```python
from build123d import *

# Parameters (mm, degrees)
SKETCH_1_R          = 3.2
SKETCH_1_R_2        = 3
SKETCH_1_W          = 46
SKETCH_1_H          = 34
EXTRUDE_1_DEPTH     = 13
SKETCH_2_R          = 11.4
EXTRUDE_2_DEPTH     = 14
SKETCH_3_R          = 1.25
CUT_EXTRUDE_1_DEPTH = 11
CUT_EXTRUDE_2_DEPTH = 14
SKETCH_5_R          = 4
EXTRUDE_3_DEPTH     = 2
SKETCH_6_R          = 1.5
EXTRUDE_4_DEPTH     = 5
EXTRUDE_5_DEPTH     = 1
SKETCH_9_W          = 26.5
SKETCH_9_H          = 7.251384336
CUT_EXTRUDE_4_DEPTH = 10


with BuildPart() as part:
    # 스케치1 → 보스-돌출1 (new body)
    with BuildSketch(Plane(origin=(0, 0, 0), x_dir=(1, 0, 0), z_dir=(0, 1, 0))):
        with BuildLine():
            Line((-61.498388188, 66.010476517), (61.501611812, 65.989522963))
            ThreePointArc((61.501611812, 65.989522963), (65.036624731, 64.524771992), (66.500805906, 60.989523028))
            Line((66.500805906, 60.989523028), (66.500805906, 4.989523158))
            ThreePointArc((66.500805906, 4.989523158), (65.03605487, 1.453704333), (61.5, -0.010476777))
            Line((61.5, -0.010476777), (-61.5, 0.010476777))
            ThreePointArc((-61.5, 0.010476777), (-65.035012919, 1.475227749), (-66.499194094, 5.010476712))
            Line((-66.499194094, 5.010476712), (-66.499194094, 61.010476582))
            ThreePointArc((-66.499194094, 61.010476582), (-65.034443058, 64.546295408), (-61.498388188, 66.010476517))
        make_face()
        with Locations((-19.054194094, 45.730282553)):
            Circle(SKETCH_1_R, mode=Mode.SUBTRACT)
        with Locations((-24.324694094, 40.396282553)):
            Circle(SKETCH_1_R, mode=Mode.SUBTRACT)
        with Locations((-13.783694094, 40.396282553)):
            Circle(SKETCH_1_R, mode=Mode.SUBTRACT)
        with Locations((-19.054194094, 35.062282553)):
            Circle(SKETCH_1_R, mode=Mode.SUBTRACT)
        with Locations((-17.339694094, 58.303282553)):
            Circle(SKETCH_1_R_2, mode=Mode.SUBTRACT)
        with Locations((43.112305906, 58.303282553)):
            Circle(SKETCH_1_R_2, mode=Mode.SUBTRACT)
        with Locations((50.675805906, 42.811282553)):
            Circle(SKETCH_1_R_2, mode=Mode.SUBTRACT)
        with Locations((43.048805906, 37.919782553)):
            Circle(SKETCH_1_R_2, mode=Mode.SUBTRACT)
        with Locations((15.743805906, 36.713282553)):
            Rectangle(SKETCH_1_W, SKETCH_1_H, mode=Mode.SUBTRACT)
    extrude(amount=EXTRUDE_1_DEPTH)

    # 스케치2 → 보스-돌출2 (add)
    with BuildSketch(Plane(origin=(0, 13, 0), x_dir=(1, 0, 0), z_dir=(0, 1, 0))):
        with BuildLine():
            ThreePointArc((-59.454194094, 37.696962121), (-55.060795812, 27.090360404), (-44.454194094, 22.696962121))
            ThreePointArc((-44.454194094, 22.696962121), (-33.847592376, 27.090360404), (-29.454194094, 37.696962121))
            Line((-29.454194094, 37.696962121), (-29.454194094, 41.666282553))
            ThreePointArc((-29.454194094, 41.666282553), (-44.454194094, 56.666282553), (-59.454194094, 41.666282553))
            Line((-59.454194094, 41.666282553), (-59.454194094, 37.696962121))
        make_face()
        with Locations((-44.454194094, 41.666282553)):
            Circle(SKETCH_2_R, mode=Mode.SUBTRACT)
    extrude(amount=EXTRUDE_2_DEPTH)

    # 스케치3 → 컷-돌출1 (cut)
    with BuildSketch(Plane.XZ):
        with Locations((-60.440145734, -59.928842317)):
            Circle(SKETCH_3_R)
        with Locations((-60.440145734, -6.092110978)):
            Circle(SKETCH_3_R)
        with Locations((60.442726529, -59.928842317)):
            Circle(SKETCH_3_R)
        with Locations((60.442726529, -6.092110978)):
            Circle(SKETCH_3_R)
        with BuildLine():
            Line((-56.500826452, -64.009622683), (56.500826452, -63.990377307))
            Line((56.500826452, -63.990377307), (56.500826452, -60.989502488))
            ThreePointArc((56.500826452, -60.989502488), (57.965286528, -57.453983111), (61.500805906, -55.989523034))
            Line((61.500805906, -55.989523034), (64.500805906, -55.989523034))
            Line((64.500805906, -55.989523034), (64.500805906, -9.989482066))
            Line((64.500805906, -9.989482066), (61.500805906, -9.989482066))
            ThreePointArc((61.500805906, -9.989482066), (57.965286528, -8.52502199), (56.500826452, -4.989502612))
            Line((56.500826452, -4.989502612), (56.500826452, -1.990377339))
            Line((56.500826452, -1.990377339), (-56.500826452, -2.009622715))
            Line((-56.500826452, -2.009622715), (-56.500826452, -4.989502612))
            ThreePointArc((-56.500826452, -4.989502612), (-57.965286528, -8.52502199), (-61.500805906, -9.989482066))
            Line((-61.500805906, -9.989482066), (-64.499194094, -9.989482066))
            Line((-64.499194094, -9.989482066), (-64.499194094, -55.989523034))
            Line((-64.499194094, -55.989523034), (-61.500805906, -55.989523034))
            ThreePointArc((-61.500805906, -55.989523034), (-57.965286528, -57.453983111), (-56.500826452, -60.989502488))
            Line((-56.500826452, -60.989502488), (-56.500826452, -64.009622683))
        make_face()
    extrude(amount=-CUT_EXTRUDE_1_DEPTH, mode=Mode.SUBTRACT)

    # 스케치4 → 컷-돌출2 (cut)
    with BuildSketch(Plane.XZ.offset(-11)):
        with BuildLine():
            Line((-31.454194094, -41.666282553), (-31.454194094, -37.696962121))
            ThreePointArc((-31.454194094, -37.696962121), (-35.261805939, -28.504573966), (-44.454194094, -24.696962121))
            ThreePointArc((-44.454194094, -24.696962121), (-53.646582249, -28.504573966), (-57.454194094, -37.696962121))
            Line((-57.454194094, -37.696962121), (-57.454194094, -41.666282553))
            ThreePointArc((-57.454194094, -41.666282553), (-44.454194094, -54.666282553), (-31.454194094, -41.666282553))
        make_face()
    extrude(amount=-CUT_EXTRUDE_2_DEPTH, mode=Mode.SUBTRACT)

    # 스케치5 → 보스-돌출3 (add)
    with BuildSketch(Plane.XZ.offset(-11)):
        with Locations((-26.039194094, -58.176282553)):
            Circle(SKETCH_5_R)
        with Locations((52.065805906, -58.176282553)):
            Circle(SKETCH_5_R)
        with Locations((-26.039194094, -11.821282553)):
            Circle(SKETCH_5_R)
        with Locations((52.065805906, -11.821282553)):
            Circle(SKETCH_5_R)
    extrude(amount=EXTRUDE_3_DEPTH)

    # 스케치6 → 보스-돌출4 (add)
    with BuildSketch(Plane.XZ.offset(-9)):
        with Locations((-26.039194094, -58.176282553)):
            Circle(SKETCH_6_R)
        with Locations((52.065805906, -58.176282553)):
            Circle(SKETCH_6_R)
        with Locations((52.065805906, -11.821282553)):
            Circle(SKETCH_6_R)
        with Locations((-26.039194094, -11.821282553)):
            Circle(SKETCH_6_R)
    extrude(amount=EXTRUDE_4_DEPTH)

    # 스케치8 → 보스-돌출5 (add)
    with BuildSketch(Plane.XZ):
        with BuildLine():
            Line((61.501611812, -65.989522963), (-61.498388188, -66.010476517))
            ThreePointArc((-61.498388188, -66.010476517), (-65.034443058, -64.546295408), (-66.499194094, -61.010476582))
            Line((-66.499194094, -61.010476582), (-66.499194094, -5.010476712))
            ThreePointArc((-66.499194094, -5.010476712), (-65.035012919, -1.475227749), (-61.5, -0.010476777))
            Line((-61.5, -0.010476777), (61.5, 0.010476777))
            ThreePointArc((61.5, 0.010476777), (65.03605487, -1.453704333), (66.500805906, -4.989523158))
            Line((66.500805906, -4.989523158), (66.500805906, -60.989523028))
            ThreePointArc((66.500805906, -60.989523028), (65.036624731, -64.524771992), (61.501611812, -65.989522963))
        make_face()
        with BuildLine():
            Line((-64.499194094, -5.010474033), (-64.499194094, -61.010473914))
            ThreePointArc((-64.499194094, -61.010473914), (-63.620333788, -63.131974892), (-61.498683162, -64.010473871))
            Line((-61.498683162, -64.010473871), (61.501316838, -63.989525671))
            ThreePointArc((61.501316838, -63.989525671), (63.622306883, -63.110665409), (64.500805906, -60.989525714))
            Line((64.500805906, -60.989525714), (64.500805906, -4.989525834))
            ThreePointArc((64.500805906, -4.989525834), (63.6219456, -2.868024856), (61.500294974, -1.989525877))
            Line((61.500294974, -1.989525877), (-61.499705026, -2.010474077))
            ThreePointArc((-61.499705026, -2.010474077), (-63.620695072, -2.889334339), (-64.499194094, -5.010474033))
        make_face(mode=Mode.SUBTRACT)
    extrude(amount=EXTRUDE_5_DEPTH)

    # 스케치9 → 컷-돌출4 (cut)
    with BuildSketch(Plane.XZ.offset(1)):
        with Locations((6.750805906, -65.426001526)):
            Rectangle(SKETCH_9_W, SKETCH_9_H)
    extrude(amount=-CUT_EXTRUDE_4_DEPTH, mode=Mode.SUBTRACT)


solid = part.part
```
CAD build for the part. Positions are in the model's coordinates, mm. A direction names the side the tool comes from. Round coordinates to 2 decimals unless told otherwise and drop trailing zeros. Write each loop counter-clockwise with the first axis right and the second up, starting at its lowest first coordinate (ties: lowest second). Pieces come first, ordered by that corner, then holes. Notation, with made-up numbers: (6, 54.25) -> (17, 54.25) arc R26 cw to (17, 87.25) -> close; hole circle Ø5 at (4, 9.5). An arc over 180 degrees is marked (long way). Answer in a Markdown table with one row per item. Add a question column.
Item 1: Saw through at B-B, the plane x = 27.5. Write the cut outline in (y, z), then the cut area to 3 significant figures.
Item 2: Drill centre lines: line 1 (Z direction, x = 54, y = 6); line 2 (X direction, y = 3.75, z = -37); line 3 (X direction, y = 15, z = -40). Where is each one in solid material? Low to high. Write a range as from..to.
Item 3: Saw through at A-A, the plane y = 15. Write the cut outline in (x, z), then the cut area to 3 significant figures.
Item 4: Mould opens along X. For faces 1 (the face through (59.194, 5.423, -6.037)), 2 (the face through (-44.124, 19.902, -56.663)), 3 (the face through (-29.454, 20, -40)) say: pulls with the +X half, pulls with the -X half, needs draft (parallel to the pull), parting line crosses it, or undercut.
Item 5: Drop flat-ended pins along their axis: pin 1 Ø12 at (x, y) = (12.5, 4.5) entering from -Z; pin 2 Ø2 at (x, z) = (-23.5, -52.5) entering from +Y; pin 3 Ø2.5 at (y, z) = (8, -4) entering from -X; pin 4 Ø10 at (y, z) = (20, -58) entering from +X. Give the stop position or say it passes through.
Item 6: Saw through at D-D, the plane x = 11. Write the cut outline in (y, z), then the cut area to 3 significant figures.
Item 7: Saw through at C-C, the plane y = 2.5. Count the separate pieces of the cut face and the enclosed holes in it, then the cut area to 3 significant figures.
Item 8: Which spindle directions (+Z, -Z, +X, -X, +Y, -Y) get a long thin tool onto all of the face, cutting with end or side? Do faces 4 (the face through (-21.594, 11.986, -33.115)), 5 (the face through (63, 5, -9.989)). Say none if no direction does.
Findings below:
| question | item | result |
|---|---|---|
| 1 | outline | (-1, -66) -> (13, -66) -> (13, -53.71) -> (11, -53.71) -> (11, -64) -> (-1, -64) -> close; (-1, -2) -> (11, -2) -> (11, -19.71) -> (13, -19.71) -> (13, 0) -> (-1, 0) -> close |
| 1 | area | 112 mm^2 |
| 2 | line 1 | z = -65.99..-63.99, -1.99..0.01 |
| 2 | line 2 | x = -66.5..-64.5, 64.5..66.5 |
| 2 | line 3 | x = -59.45..-57.45, -31.45..-29.45 |
| 3 | outline | (-59.45, -41.67) arc R15 ccw to (-29.45, -41.67) -> (-29.45, -37.7) arc R15 ccw to (-59.45, -37.7) -> close; hole (-57.45, -41.67) arc R13 ccw to (-31.45, -41.67) -> (-31.45, -37.7) arc R13 ccw to (-57.45, -37.7) -> close |
| 3 | area | 192 mm^2 |
| 4 | face 1 | undercut |
| 4 | face 2 | parting line crosses it |
| 4 | face 3 | pulls with the +X half |
| 5 | pin 1 | stops at z = -66 |
| 5 | pin 2 | stops at y = 13 |
| 5 | pin 3 | stops at x = -66.5 |
| 5 | pin 4 | stops at x = -34.63 |
| 6 | outline | (-1, -2) -> (11, -2) -> (11, -19.71) -> (13, -19.71) -> (13, 0) -> (-1, 0) -> close; (9, -66) -> (13, -66) -> (13, -53.71) -> (11, -53.71) -> (11, -64) -> (9, -64) -> close |
| 6 | area | 92.0 mm^2 |
| 7 | separate pieces | 1 |
| 7 | enclosed holes | 4 |
| 7 | area | 920 mm^2 |
| 8 | face 4 | +Y, -Y |
| 8 | face 5 | -Y |
